The model under review builds one solid part; all positions refer to its coordinate system, in mm. A direction names the side the tool comes from. Round coordinates to 2 decimals unless told otherwise and drop trailing zeros. Order: outer loops, then holes, each group sorted by start corner. A loop starts at its lowest first (then second) coordinate and runs counter-clockwise, first axis right, second up. Notation, with made-up numbers: M 34,-10 L 44,-10 A8 cw 44,-1 Z; hole C 31,55.5 d5. An arc over 180 degrees is marked long. Answer as a JSON object with one key per item and string values. Group by question number.
1) The part is to be moulded in two halves that separate along Z. For faces 4 (the cylindrical face through (28.543, -8.874, -13.413)), 5 (the flat face through (-1, -9, -41.098)), 6 (the flat face through (-45.45, -6.87, -35.098)), 7 (the cylindrical face through (43.526, -10.352, -38.14)), say which applies: +Z half, -Z half, draft (parallel to the pull), parting line (faces both ways), or undercut.
2) For faces 1 (the cylindrical face through (-28.16, -8.87, -14.37)), 2 (the flat face through (33.074, -9, -15)), 3 (the cylindrical face through (51.4, -0.57, -38.06)), list the 3-axis set-ups (+Z, -Z, +X, -X, +Y, -Y) from which the entire face can be reached by the end or side of a thin tool; tool diameter is ignored.
3) Consider section B-B, the plane x = 45. Write out the cut boundary in (y, z), then the cut area to 3 significant figures.
4) Insertion check: pin 1 Ø1.5 at (x, z) = (27.5, -15.5) entering from -Y; pin 2 Ø6.5 at (x, y) = (47, -8) entering from +Z; pin 3 Ø1.5 at (y, z) = (-12.5, 12) entering from -X; pin 4 Ø5.5 at (y, z) = (-5.5, -10) entering from -X. Each pin has a flat end and moves straight along its axis. Give the tip position at first contact, or say it passes through.
5) Consider section A-A, the plane z = -7. Write out the cut boundary in (x, y), then the cut area to 3 significant figures.
6) To check wall thickness, follow line 1 (X direction, y = -9, z = -37.75); line 2 (Y direction, x = -45, z = -36); line 3 (Z direction, x = 41, y = -16.75). State the ranges of each line that lie inside material, in increasing order.
7) Consider section D-D, the plane x = -17.5. Write out the cut boundary in (y, z).
8) Consider section C-C, the plane y = -9. Write out the cut boundary in (x, z), then the cut area to 3 significant figures.
```python
from build123d import *

# Parameters (mm, degrees)
F1_DEPTH = 18
F2_R     = 2
F3_DEPTH = 6
F4_R     = 2
F5_R     = 6


with BuildPart() as f1:
    # F0 (on Front) → F1 (new body)
    with BuildSketch(Plane.XZ):
        with BuildLine():
            ThreePointArc((21.663506, 20.276783), (28.356264, -13.893308), (0, -34.1))
            ThreePointArc((0, -34.1), (-28.356264, -13.893308), (-21.663506, 20.276783))
            ThreePointArc((-21.663506, 20.276783), (-21.384271, 20.979731), (-21.677117, 21.677117))
            Line((-21.677117, 21.677117), (-22.384578, 22.384578))
            ThreePointArc((-22.384578, 22.384578), (-23.107247, 22.67735), (-23.820455, 22.362229))
            ThreePointArc((-23.820455, 22.362229), (-30.676458, 11.564077), (-33.074125, -1))
            Line((-33.074125, -1), (-33.074125, -35.098328))
            Line((-33.074125, -35.098328), (-52, -35.098328))
            Line((-52, -35.098328), (-52, -41.098328))
            Line((-52, -41.098328), (0, -41.098328))
            Line((0, -41.098328), (52, -41.098328))
            Line((52, -41.098328), (52, -35.098328))
            Line((52, -35.098328), (33.074125, -35.098328))
            Line((33.074125, -35.098328), (33.074125, -1))
            ThreePointArc((33.074125, -1), (30.676458, 11.564077), (23.820455, 22.362229))
            ThreePointArc((23.820455, 22.362229), (23.107247, 22.67735), (22.384578, 22.384578))
            Line((22.384578, 22.384578), (21.677117, 21.677117))
            ThreePointArc((21.677117, 21.677117), (21.384271, 20.979731), (21.663506, 20.276783))
        make_face()
    extrude(amount=F1_DEPTH)

    # F2 (on face) → F3 (cut, through all)
    with BuildSketch(Plane(origin=(0, 0, -41.098328), x_dir=(1, 0, 0), z_dir=(0, 0, -1))):
        with Locations((-45, 9)):
            Circle(F2_R)
        with Locations((45, 9)):
            Circle(F2_R)
    extrude(amount=-F3_DEPTH, mode=Mode.SUBTRACT)

    # F4
    f4_edges = [f1.edges().sort_by_distance(p)[0] for p in [
        (-52, 0, -38.098328),
        (-52, -18, -38.098328),
        (52, -18, -38.098328),
        (52, 0, -38.098328),
    ]]
    fillet(f4_edges, radius=F4_R)

    # F5
    f5_edges = [f1.edges().sort_by_distance(p)[0] for p in [
        (-33.074125, -9, -35.098328),
        (33.074125, -9, -35.098328),
    ]]
    fillet(f5_edges, radius=F5_R)


solid = f1.part
```
Results list:
{
 "1": {"face 4": "undercut", "face 5": "-Z half", "face 6": "+Z half", "face 7": "draft"},
 "2": {"face 1": "+Y, -Y", "face 2": "+Z, +X, +Y, -Y", "face 3": "+Z, -Z, +X, +Y"},
 "3": {"outline": "M -18,-41.1 L -11,-41.1 L -11,-35.1 L -18,-35.1 Z; M -7,-41.1 L 0,-41.1 L 0,-35.1 L -7,-35.1 Z", "area": "84.0 mm^2"},
 "4": {"pin 1": "y = -18", "pin 2": "z = -35.1", "pin 3": "x = -30.8", "pin 4": "x = -33.07"},
 "5": {"outline": "M -33.07,-18 L -30.25,-18 L -30.25,0 L -33.07,0 Z; M 30.25,-18 L 33.07,-18 L 33.07,0 L 30.25,0 Z", "area": "102 mm^2"},
 "6": {"line 1": "-52 to -47, -43 to 43, 47 to 52", "line 2": "-18 to -11, -7 to 0", "line 3": "-41.1 to -35.1"},
 "7": {"outline": "M -18,-41.1 L 0,-41.1 L 0,-27.92 L -18,-27.92 Z"},
 "8": {"outline": "M -52,-41.1 L -47,-41.1 L -47,-35.1 L -52,-35.1 Z; M -43,-41.1 L 43,-41.1 L 43,-35.1 L 39.07,-35.1 A6 cw 33.07,-29.1 L 33.07,-1 A34.12 ccw 23.82,22.36 A1 ccw 22.38,22.38 L 21.68,21.68 A1 ccw 21.66,20.28 A32.13 cw 0,-34.1 A32.13 cw -21.66,20.28 A1 ccw -21.68,21.68 L -22.38,22.38 A1 ccw -23.82,22.36 A34.12 ccw -33.07,-1 L -33.07,-29.1 A6 cw -39.07,-35.1 L -43,-35.1 Z; M 47,-41.1 L 52,-41.1 L 52,-35.1 L 47,-35.1 Z", "area": "1,400 mm^2"}
}
